Part model, mm, in its own coordinate system. A direction names the side the tool comes from. Round coordinates to 2 decimals unless told otherwise and drop trailing zeros. Loops run counter-clockwise (first coordinate to the right, second up) from the corner with the lowest first, then second, coordinate; pieces in that order, holes last. Notation, with made-up numbers: (44, 17) -> (97, 17) arc R12 ccw to (97, 34) -> close; hole circle Ø9 at (-23.75, -3). An arc over 180 degrees is marked (long way). Use a Markdown table: item, result. Add a question column.
Item 1: Cut at A-A, the plane z = 36.1. List the corners of the cut face in (x, y), plus the area to 3 significant figures.
Item 2: Cut at B-B, the plane x = 5. List the corners of the cut face in (y, z), plus the area to 4 significant figures.
Item 3: Cut at C-C, the plane z = 22. List the corners of the cut face in (x, y).
Item 4: Probe line 1 (X direction, y = 3.95, z = 10); line 2 (X direction, y = 8.75, z = 5); line 3 (Y direction, x = 7, z = 6). List the from-to ranges inside material, lowest first. Write a range as [from, to].
Item 5: Cut at D-D, the plane y = 6.5. List the corners of the cut face in (x, z), plus the area to 3 significant figures.
Item 6: Which spindle directions (+Z, -Z, +X, -X, +Y, -Y) get a long thin tool onto all of the face, cutting with end or side? Do faces 1 (the face through (55, 5, 23)), 2 (the face through (4, 5, 23)), 3 (the face through (53.925, 2.465, 34.714)). Say none if no direction does.
Item 7: Two-plate mould, pull along Z, no slides. Class faces 4 (the face through (5.07, 2.46, 11.5)), 5 (the face through (30, 6, 46.1)), 6 (the face through (51.5, 8, 23)): pulls with the +Z half, pulls with the -Z half, needs draft (parallel to the pull), parting line crosses it, or undercut.
Item 8: Flat gauge pins, fed straight in: pin 1 (5 mm diameter, centred on x = 5, z = 10, fed in from +Y); pin 2 (3 mm diameter, centred on y = 10.5, z = 6, fed in from +X); pin 3 (5.5 mm diameter, centred on y = 9.5, z = 18.5, fed in from -X). Where does each tip first touch, or does it go through?
```python
from build123d import *

# Parameters (mm, degrees)
EXTRUDE_1_DEPTH     = 46.1
SKETCH_2_R          = 1.5
CUT_EXTRUDE_1_DEPTH = 77.173158002


with BuildPart() as part:
    # 草图1 → 凸台-拉伸1 (new body)
    with BuildSketch(Plane.XY):
        Polygon((0, 0), (0, 5), (8, 5), (8, 11.7), (51.5, 11.7), (51.5, 5), (59.5, 5), (59.5, 0), align=None)
    extrude(amount=EXTRUDE_1_DEPTH)

    # 草图2 → 切除-拉伸1 (cut, through all)
    with BuildSketch(Plane.XZ):
        with Locations(Location((5, 36.1, 0), (0, 0, 270))):
            Circle(SKETCH_2_R)
        with Locations(Location((5, 10, 0), (0, 0, 270))):
            Circle(SKETCH_2_R)
        with Locations(Location((54.5, 36.1, 0), (0, 0, 270))):
            Circle(SKETCH_2_R)
        with Locations(Location((54.5, 10, 0), (0, 0, 270))):
            Circle(SKETCH_2_R)
    extrude(amount=-CUT_EXTRUDE_1_DEPTH, mode=Mode.SUBTRACT)


solid = part.part
```
A:
| question | item | result |
|---|---|---|
| 1 | outline | (0, 0) -> (3.5, 0) -> (3.5, 5) -> (0, 5) -> close; (6.5, 0) -> (53, 0) -> (53, 5) -> (51.5, 5) -> (51.5, 11.7) -> (8, 11.7) -> (8, 5) -> (6.5, 5) -> close; (56, 0) -> (59.5, 0) -> (59.5, 5) -> (56, 5) -> close |
| 1 | area | 559 mm^2 |
| 2 | outline | (0, 0) -> (5, 0) -> (5, 8.5) -> (0, 8.5) -> close; (0, 11.5) -> (5, 11.5) -> (5, 34.6) -> (0, 34.6) -> close; (0, 37.6) -> (5, 37.6) -> (5, 46.1) -> (0, 46.1) -> close |
| 2 | area | 200.5 mm^2 |
| 3 | outline | (0, 0) -> (59.5, 0) -> (59.5, 5) -> (51.5, 5) -> (51.5, 11.7) -> (8, 11.7) -> (8, 5) -> (0, 5) -> close |
| 4 | line 1 | x = [0, 3.5], [6.5, 53], [56, 59.5] |
| 4 | line 2 | x = [8, 51.5] |
| 4 | line 3 | y = [0, 5] |
| 5 | outline | (8, 0) -> (51.5, 0) -> (51.5, 46.1) -> (8, 46.1) -> close |
| 5 | area | 2,010 mm^2 |
| 6 | face 1 | +Z, -Z, +X, +Y |
| 6 | face 2 | +Z, -Z, -X, +Y |
| 6 | face 3 | +Y, -Y |
| 7 | face 4 | undercut |
| 7 | face 5 | pulls with the +Z half |
| 7 | face 6 | needs draft |
| 8 | pin 1 | stops at y = 5 |
| 8 | pin 2 | stops at x = 51.5 |
| 8 | pin 3 | stops at x = 8 |
